Input: part model. Units: mm. Frame: model coordinates. A direction names the side the tool comes from. Coordinates: 2 decimals unless noted, no trailing zeros. Loops run counter-clockwise (first coordinate to the right, second up) from the corner with the lowest first, then second, coordinate; pieces in that order, holes last.
```python
from build123d import *

# Parameters (mm, degrees)
SKETCH2_W           = 20
SKETCH2_H           = 15
BOSS_EXTRUDE1_DEPTH = 50
SKETCH3_R           = 1.65
CUT_EXTRUDE1_DEPTH  = 54.150729064


with BuildPart() as part:
    # Sketch2 → Boss-Extrude1 (new body)
    with BuildSketch(Plane.XY):
        with Locations((0, 3.75)):
            Rectangle(SKETCH2_W, SKETCH2_H)
        with BuildLine():
            Line((6.18, 0.4025), (6.18, 2.9775))
            Line((6.18, 2.9775), (5.988999354, 4.060718492))
            ThreePointArc((5.988999354, 4.060718492), (4.929202717, 5.285218638), (5.905225776, 6.577483513))
            Line((5.905225776, 6.577483513), (5.722724444, 7.6125))
            Line((5.722724444, 7.6125), (-5.362724444, 7.6125))
            Line((-5.362724444, 7.6125), (-5.545225776, 6.577483513))
            ThreePointArc((-5.545225776, 6.577483513), (-4.654560018, 5.122927971), (-5.988999354, 4.060718492))
            Line((-5.988999354, 4.060718492), (-6.18, 2.9775))
            Line((-6.18, 2.9775), (-6.18, 0.4025))
            Line((-6.18, 0.4025), (-5.665, -0.1125))
            Line((-5.665, -0.1125), (5.665, -0.1125))
            Line((5.665, -0.1125), (6.18, 0.4025))
        make_face(mode=Mode.SUBTRACT)
    extrude(amount=BOSS_EXTRUDE1_DEPTH)

    # Sketch3 → Cut-Extrude1 (cut, through all)
    with BuildSketch(Plane(origin=(0, 11.25, 0), x_dir=(1, 0, 0), z_dir=(0, 1, 0))):
        with Locations(Location((0, -5, 0), (0, 0, 270))):
            Circle(SKETCH3_R)
        with Locations(Location((0, -30, 0), (0, 0, 270))):
            Circle(SKETCH3_R)
    extrude(amount=-CUT_EXTRUDE1_DEPTH, mode=Mode.SUBTRACT)


solid = part.part
```
Item 1: Section query C-C (y = 1.5). Output: boundary loops of the cut face in (x, z), then the cut area to 3 significant figures.
Result:
outline: (-10, 0) - (-6.18, 0) - (-6.18, 50) - (-10, 50) - close; (6.18, 0) - (10, 0) - (10, 50) - (6.18, 50) - close
area: 382 mm2
Item 2: Line query: L1, parallel to Y at x = -1, z = 42; L2, parallel to Z at x = -1.25, y = 10; L3, parallel to X at y = 8.95, z = 30. Output: solid intervals per line, ascending.
Result:
L1: y = -3.75 to -0.11, 7.61 to 11.25
L2: z = 0 to 3.92, 6.08 to 28.92, 31.08 to 50
L3: x = -10 to -1.65, 1.65 to 10
Item 3: Contact query for a flat-ended pin moving along its axis: P1, Ø2, axis at x = 1.5, z = 29.5, coming from the -Y side. Output: stop coordinate, or through.
Result:
P1: stops at y = -3.75
Item 4: Section query B-B (x = 0). Output: boundary loops of the cut face in (y, z).
Result:
outline: (-3.75, 0) - (-0.11, 0) - (-0.11, 3.35) - (-3.75, 3.35) - close; (-3.75, 6.65) - (-0.11, 6.65) - (-0.11, 28.35) - (-3.75, 28.35) - close; (-3.75, 31.65) - (-0.11, 31.65) - (-0.11, 50) - (-3.75, 50) - close; (7.61, 0) - (11.25, 0) - (11.25, 3.35) - (7.61, 3.35) - close; (7.61, 6.65) - (11.25, 6.65) - (11.25, 28.35) - (7.61, 28.35) - close; (7.61, 31.65) - (11.25, 31.65) - (11.25, 50) - (7.61, 50) - close
Item 5: Mould query, pull axis Y, two halves, no side actions, for faces 3 (the face through (0, 11.25, 25)), 4 (the face through (-4.65, 5.15, 24.65)), 5 (the face through (-6.18, 2, 25)), 6 (the face through (10, 4, 25)). Classes: +Y half, -Y half, draft (parallel to the pull), parting line (faces both ways), or undercut.
Result:
face 3: +Y half
face 4: undercut
face 5: undercut
face 6: draft
Item 6: Reachability of faces 1 (the face through (0, -0.112, 25)), 2 (the face through (0.07, 9.46, 3.35)) from +Z, -Z, +X, -X, +Y, -Y: full face, straight path, thin tool, end or side. Return the list, or none.
Result:
face 1: +Z, -Z
face 2: +Y, -Y
